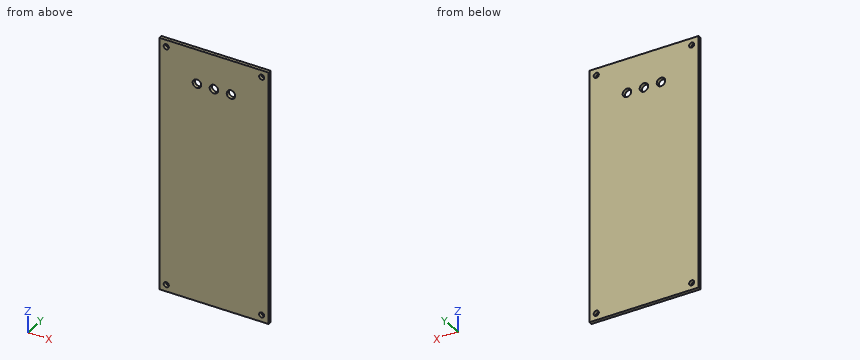
Autodesk Inventor part; units mm, degrees
ref_plane "YZ Plane" through (0, 0, 0) normal (1, 0, 0) x (0, 1, 0)
ref_plane "XZ Plane" through (0, 0, 0) normal (0, 1, 0) x (-1, 0, 0)
ref_plane "XY Plane" through (0, 0, 0) normal (0, 0, 1) x (1, 0, 0)
sketch "Sketch2" plane through (0, 0, 0) normal (0, 1, 0) x (-1, 0, 0)
  line L0 (0, 0) -> (64, 0)
  line L1 (64, 0) -> (64, -148)
  line L2 (64, -148) -> (0, -148)
  line L3 (0, -148) -> (0, 0)
  dimension "d0" = 64
  dimension "d1" = 148
extrude "Extrusion1" add sketch "Sketch2" along normal blind 2
sketch "Sketch3" plane through (0, 2, 0) normal (0, 1, 0) x (1, 0, 0)
  circle A0 centre (-4, 4) radius 1.5
  circle A1 centre (-60, 4) radius 1.5
  circle A2 centre (-60, 144) radius 1.5
  circle A3 centre (-4, 144) radius 1.5
  line L0 (0, 0) -> (0, 148)
  line L1 (-64, 0) -> (0, 0)
  line L2 (-64, 148) -> (-64, 0)
  line L3 (0, 148) -> (-64, 148)
  point P0 (0, 0.5)
  point P1 (0, 147.5)
  point P2 (-63.5, 0)
  point P3 (-0.5, 0)
  point P4 (-64, 147.5)
  point P5 (-64, 0.5)
  point P6 (-0.5, 148)
  point P7 (-63.5, 148)
  dimension "d10" = 3
  dimension "d11" = 3
  dimension "d12" = 3
  dimension "d13" = 3
  dimension "d14" = 4
  dimension "d15" = 4
  dimension "d16" = 4
  dimension "d17" = 4
  dimension "d18" = 4
  dimension "d19" = 4
  dimension "d20" = 4
  dimension "d21" = 4
extrude "Extrusion2" cut sketch "Sketch3" against normal blind 2 contours A0 | A1 | A2 | A3
sketch "Sketch4" plane through (0, 2, 0) normal (0, 1, 0) x (1, 0, 0)
  circle A0 centre (-22, 20) radius 2.5
  circle A1 centre (-32, 20) radius 2.5
  circle A2 centre (-42, 20) radius 2.5
  line L0 (0, 0) -> (0, 148)
  line L1 (-64, 0) -> (0, 0)
  point P0 (0, 0.5)
  point P1 (0, 147.5)
  point P2 (-63.5, 0)
  point P3 (-0.5, 0)
  point P4 (-32, 0)
  dimension "d24" = 5
  dimension "d25" = 5
  dimension "d26" = 5
  dimension "d28" = 32
  dimension "d29" = 10
  dimension "d30" = 10
  dimension "d31" = 20
extrude "Extrusion3" cut sketch "Sketch4" against normal blind 2
properties part number "kotelo_kansi"
Part model, mm, in its own coordinate system. Round coordinates to 2 decimals unless told otherwise and drop trailing zeros. Write each loop counter-clockwise with the first axis right and the second up, starting at its lowest first coordinate (ties: lowest second). Pieces come first, ordered by that corner, then holes. Notation, with made-up numbers: M -8.5,7.25 L 22.5,7.25 A20 ccw 22.5,26.25 Z; hole C 13,42.5 d1. An arc over 180 degrees is marked long. Return JSON: item names as keys, results as strings. Group by question number.
(1) Drill centre lines: probe 1 along X at (y, z) = (0.8, -144); probe 2 along Z at (x, y) = (-60, 1.6); probe 3 along Z at (x, y) = (-22, 1.4). Where is each one in solid material? Low to high.
(2) Saw through at C-C on x = -32. Write the cut outline in (y, z), then the cut area to 3 significant figures.
(3) Saw through at B-B on x = -4. Write the cut outline in (y, z), then the cut area to 3 significant figures.
(4) Saw through at A-A on z = -144. Write the cut outline in (x, y).
(5) Pin check, flat tip, straight feed: pin 1 Ø4 at (x, z) = (-32, -20) entering from +Y. Stop position of the tip, or through.
Returned:
{
 "1": {"probe 1": "-64 to -61.5, -58.5 to -5.5, -2.5 to 0", "probe 2": "-148 to -145.5, -142.5 to -5.5, -2.5 to 0", "probe 3": "-148 to -22.5, -17.5 to 0"},
 "2": {"outline": "M 0,-148 L 2,-148 L 2,-22.5 L 0,-22.5 Z; M 0,-17.5 L 2,-17.5 L 2,0 L 0,0 Z", "area": "286 mm²"},
 "3": {"outline": "M 0,-148 L 2,-148 L 2,-145.5 L 0,-145.5 Z; M 0,-142.5 L 2,-142.5 L 2,-5.5 L 0,-5.5 Z; M 0,-2.5 L 2,-2.5 L 2,0 L 0,0 Z", "area": "284 mm²"},
 "4": {"outline": "M -64,0 L -61.5,0 L -61.5,2 L -64,2 Z; M -58.5,0 L -5.5,0 L -5.5,2 L -58.5,2 Z; M -2.5,0 L 0,0 L 0,2 L -2.5,2 Z"},
 "5": {"pin 1": "through"}
}
